The model under review builds one solid part; all positions refer to its coordinate system, in mm. Face numbers are marked on the shaded views. A direction names the side the tool comes from. Give positions to 0.01 mm unless a question says otherwise; leave off trailing zeros. Order: outer loops, then holes, each group sorted by start corner. A loop starts at its lowest first (then second) coordinate and runs counter-clockwise, first axis right, second up.
Autodesk Inventor part; units mm, degrees
ref_plane "YZ Plane" through (0, 0, 0) normal (1, 0, 0) x (0, 1, 0)
ref_plane "XZ Plane" through (0, 0, 0) normal (0, 1, 0) x (-1, 0, 0)
ref_plane "XY Plane" through (0, 0, 0) normal (0, 0, 1) x (1, 0, 0)
sketch "Sketch1" plane through (0, 0, 0) normal (1, 0, 0) x (0, 1, 0)
  line L0 (0, 58.45) -> (0, -119.35)
  line L1 (0, -119.35) -> (50.8, -119.35)
  line L2 (50.8, -119.35) -> (50.8, 58.45)
  line L3 (50.8, 58.45) -> (0, 58.45)
  point P0 (0, 0)
  dimension "d0" = 177.8
  dimension "d1" = 50.8
  dimension "d2" = 177.8
extrude "Extrusion1" add sketch "Sketch1" along normal blind 127
sketch "Sketch2" plane through (0, 50.8, 58.45) normal (0, 1, 0) x (1, 0, 0)
  line L0 (0, 0) -> (0, 50.8)
  line L1 (0, 0) -> (0, 177.8)
  line L2 (0, 50.8) -> (127, 50.8)
  line L3 (127, 0) -> (127, 177.8)
  line L4 (127, 50.8) -> (127, 0)
  line L5 (0, 0) -> (127, 0)
  line L6 (127, 0) -> (0, 0)
  point P0 (0, 58.45)
  dimension "d5" = 50.8
extrude "Extrusion2" add sketch "Sketch2" along normal blind 76.2
sketch "Sketch3" plane through (0, 50.8, -119.35) normal (0, 1, 0) x (1, 0, 0)
  line L0 (0, 0) -> (127, 0)
  line L1 (50.7885, 0) -> (50.7885, -76.1988)
  line L2 (50.7885, -76.1988) -> (76.1885, -76.1988)
  line L3 (76.1885, -76.1988) -> (76.1885, 0)
  line L4 (50.7885, 0) -> (76.1885, 0)
  point P0 (0, -119.35)
  dimension "d8" = 25.4
extrude "Extrusion3" cut sketch "Sketch3" against normal blind 50.8
sketch "Sketch4" plane through (127, 50.8, 7.65) normal (0, 0, -1) x (-1, 0, 0)
  line L0 (0, 76.2) -> (127, 76.2)
  line L1 (25.3885, 76.2) -> (25.3745, 50.7949)
  line L2 (25.3745, 50.7949) -> (101.5745, 50.7531)
  line L3 (101.5745, 50.7531) -> (101.5885, 76.2)
  line L4 (25.3885, 76.2) -> (101.5885, 76.2)
  point P0 (127, -50.8)
  dimension "d11" = 76.2
extrude "Extrusion4" cut sketch "Sketch4" against normal blind 50.8
properties part number "AddSub (1)"
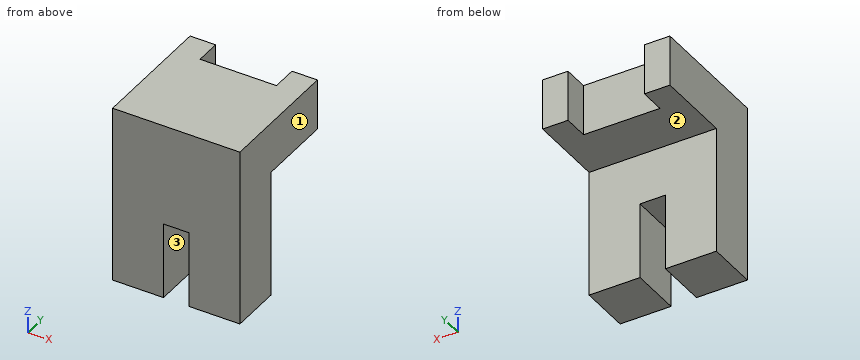
1. Take a section at B-B (y = 23.5). Write out the cut boundary in (x, z).
2. Take a section at D-D (z = 20). Write out the cut boundary in (x, y).
3. Take a section at C-C (x = 116.5). Write out the cut boundary in (y, z).
4. Take a section at A-A (z = -62). Write out the cut boundary in (x, y), and give its area (3 significant figures).
5. Insertion check: pin 1 (1.5 mm diameter, centred on x = 113.5, z = -57.5, fed in from +Y); pin 2 (12.5 mm diameter, centred on x = 64.5, y = 21, fed in from -Z). Each pin has a flat end and moves straight along its axis. Give the tip position at first contact, or say it passes through.
6. For the marked faces 1, 2 and 3, list the 3-axis set-ups (+Z, -Z, +X, -X, +Y, -Y) from which the entire face can be reached by the end or side of a thin tool; tool diameter is ignored.
7. To check wall thickness, follow line 1 (Z direction, x = 115, y = 104.5); line 2 (Y direction, x = 102.5, z = -109); line 3 (X direction, y = 38, z = -81.5). State the ranges of each line that lie inside material, in increasing order.
Answer:
1. outline: (0, -119.35) - (50.79, -119.35) - (50.79, -43.15) - (76.19, -43.15) - (76.19, -119.35) - (127, -119.35) - (127, 58.45) - (0, 58.45) - close
2. outline: (0, 0) - (127, 0) - (127, 127) - (101.61, 127) - (101.63, 101.59) - (25.43, 101.55) - (25.41, 127) - (0, 127) - close
3. outline: (0, -119.35) - (50.8, -119.35) - (50.8, 7.65) - (127, 7.65) - (127, 58.45) - (0, 58.45) - close
4. outline: (0, 0) - (50.79, 0) - (50.79, 50.8) - (0, 50.8) - close; (76.19, 0) - (127, 0) - (127, 50.8) - (76.19, 50.8) - close
4. area: 5,160 mm2
5. pin 1: stops at y = 50.8
5. pin 2: stops at z = -43.15
6. face 1: +Z, -Z, +X, +Y, -Y
6. face 2: -Z, +X, -X, +Y
6. face 3: -Z, +Y, -Y
7. line 1: z = 7.65 to 58.45
7. line 2: y = 0 to 50.8
7. line 3: x = 0 to 50.79, 76.19 to 127
